Can you work these out from the drawing? Everything is in mm from the part's minimum corner. A direction names the side the tool comes from. Round coordinates to 2 decimals unless told otherwise and drop trailing zeros. Order: outer loops, then holes, each group sorted by start corner. A loop starts at its lowest first (then second) coordinate and runs counter-clockwise, first axis right, second up. Notation, with made-up numbers: M 43,-15 L 61,-15 A25 ccw 61,19 Z; hole C 18,63.5 d11. An arc over 180 degrees is marked long. Write item = value, one per line. Start each with the question number.
Item 1: I want a section at D-D, the plane x = 23. List the corners of the cut face in (y, z) for me, plus the area to 3 significant figures.
Item 2: I want a section at B-B, the plane y = 9. List the corners of the cut face in (x, z) for me.
Item 3: Please list where these lines run through material, in increasing order: L1, parallel to X at y = 25, z = 10.75; L2, parallel to Z at x = 32.5, y = 38.2; L3, parallel to Y at x = 50.5, z = 3.5.
Item 4: I want a section at C-C, the plane z = 18.5. List the corners of the cut face in (x, y) for me.
Item 5: I'm going to push a flat-ended pin straight in: P1, Ø3.5, axis at x = 42.5, z = 5, coming from the -Y side. Where does the tip first touch, or does it pass through?
Item 6: We'd pull the mould along X, two halves only. Please class the marked faces 3, 4, 5 and 6: pulls with the +X half, pulls with the -X half, needs draft (parallel to the pull), parting line crosses it, or undercut.
Item 7: I want a section at A-A, the plane x = 32.5. List the corners of the cut face in (y, z) for me, plus the area to 3 significant figures.
Item 8: For the marked faces 1 and 2, which set-ups out of +Z, -Z, +X, -X, +Y, -Y let a thin tool reach every point of the face, with its end or its side?
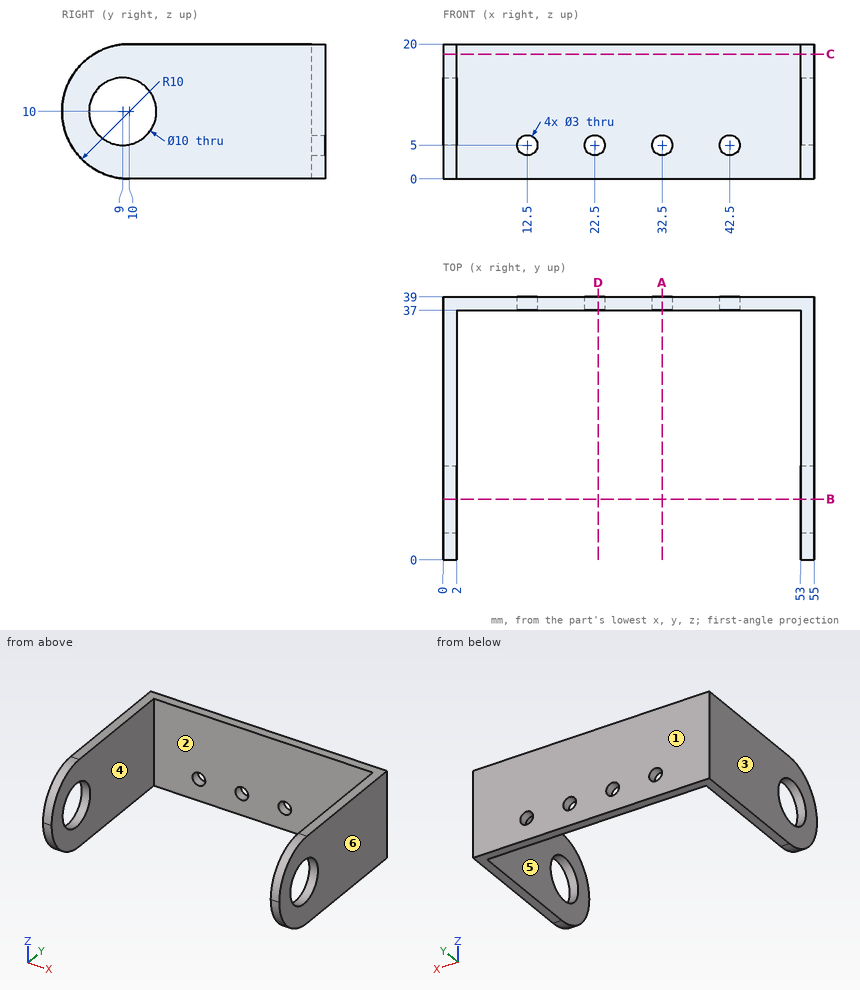
Filled in:
q1.outline = M 37,0 L 39,0 L 39,3.59 L 37,3.59 Z; M 37,6.41 L 39,6.41 L 39,20 L 37,20 Z
q1.area = 34.3 mm^2
q2.outline = M 0,0.05 L 2,0.05 L 2,5 L 0,5 Z; M 0,15 L 2,15 L 2,19.95 L 0,19.95 Z; M 53,0.05 L 55,0.05 L 55,5 L 53,5 Z; M 53,15 L 55,15 L 55,19.95 L 53,19.95 Z
q3.L1 = 0 to 2, 53 to 55
q3.L2 = 0 to 3.5, 6.5 to 20
q3.L3 = 37 to 39
q4.outline = M 0,4.73 L 2,4.73 L 2,37 L 53,37 L 53,4.73 L 55,4.73 L 55,39 L 0,39 Z
q5.P1 = 37
q6.face_3 = pulls with the -X half
q6.face_4 = undercut
q6.face_5 = undercut
q6.face_6 = pulls with the +X half
q7.outline = M 37,0 L 39,0 L 39,3.5 L 37,3.5 Z; M 37,6.5 L 39,6.5 L 39,20 L 37,20 Z
q7.area = 34.0 mm^2
q8.face_1 = +Z, -Z, +X, -X, +Y
q8.face_2 = +Z, -Z, -Y
